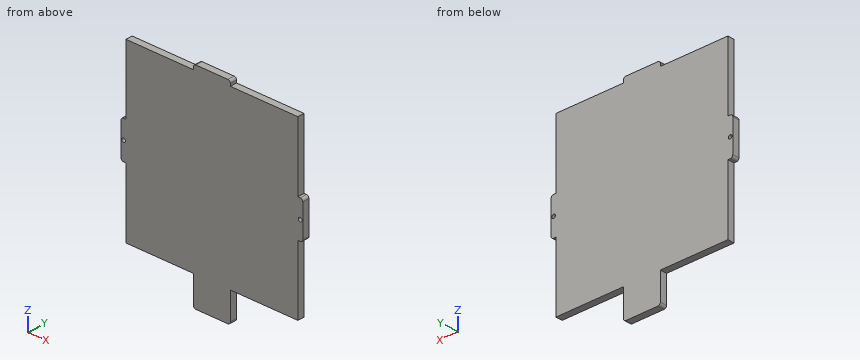
from build123d import *

# Parameters (mm, degrees)
SKETCH1_R           = 1.5
BOSS_EXTRUDE1_DEPTH = 5.5
FILLET1_R           = 2


with BuildPart() as part:
    # Sketch1 → Boss-Extrude1 (new body)
    with BuildSketch(Plane(origin=(0, 0, 0), x_dir=(1, 0, 0), z_dir=(0, 1, 0))):
        Polygon((0, 85), (0, 140), (55, 140), (55, 164), (85, 164), (85, 140), (140, 140), (140, 85), (144, 85), (144, 55), (140, 55), (140, 0), (85, 0), (85, -4), (55, -4), (55, 0), (0, 0), (0, 55), (-4, 55), (-4, 85), align=None)
        with Locations(Location((-1.9, 70, 0), (0, 0, 270))):
            Circle(SKETCH1_R, mode=Mode.SUBTRACT)
        with Locations(Location((141.9, 70, 0), (0, 0, 270))):
            Circle(SKETCH1_R, mode=Mode.SUBTRACT)
    extrude(amount=BOSS_EXTRUDE1_DEPTH)

    # Fillet1
    fillet1_edges = [part.edges().sort_by_distance(p)[0] for p in [
        (-4, 2.75, -55),
        (-4, 2.75, -85),
        (55, 2.75, -164),
        (85, 2.75, -164),
        (144, 2.75, -85),
        (144, 2.75, -55),
        (85, 2.75, 4),
        (55, 2.75, 4),
    ]]
    fillet(fillet1_edges, radius=FILLET1_R)


solid = part.part
Check sheet for the modelled part. Datum: model origin and axes. Units: mm. Round coordinates to 2 decimals unless told otherwise and drop trailing zeros. Order: outer loops, then holes, each group sorted by start corner. A loop starts at its lowest first (then second) coordinate and runs counter-clockwise, first axis right, second up.
(1) Scan lines: probe 1 along X at (y, z) = (3.1, -70); probe 2 along X at (y, z) = (4.9, -126); probe 3 along Z at (x, y) = (96, 3.25). Record each from-to range of solid material in increasing order.
(2) Cross-section at C-C, the plane x = 88. Enter the section's corners in (y, z).
(3) Go/stop test with flat-tipped pins: P1, Ø0.6, axis at x = 141, y = 2, coming from the -Z side; P2, Ø1.5, axis at y = 1.5, z = -136, coming from the +X side; P3, Ø3, axis at y = 2, z = -147.5, coming from the +X side; P4, Ø2.5, axis at x = -1.9, z = -70, coming from the -Y side. Record where each tip stops, or that it passes through.
(4) Cross-section at A-A, the plane y = 3.4. State how many separate pieces and enclosed holes the cut face has, and give its area (3 significant figures).
(5) Cross-section at B-B, the plane z = -47. Enter the section's corners in (x, y).
Check sheet entries:
1. probe 1: x = -4 to -3.4, -0.4 to 140.4, 143.4 to 144
1. probe 2: x = 0 to 140
1. probe 3: z = -140 to 0
2. outline: (0, -140) - (5.5, -140) - (5.5, 0) - (0, 0) - close
3. P1: stops at z = -85
3. P2: stops at x = 140
3. P3: stops at x = 85
3. P4: passes through
4. separate pieces: 1
4. enclosed holes: 2
4. area: 20,700 mm2
5. outline: (0, 0) - (140, 0) - (140, 5.5) - (0, 5.5) - close
